Design review of the part built by this model. Coordinates are the model's own, in mm. Face numbers are marked on the shaded views. Coordinates: 2 decimals unless noted, no trailing zeros. Loops run counter-clockwise (first coordinate to the right, second up) from the corner with the lowest first, then second, coordinate; pieces in that order, holes last. Notation, with made-up numbers: (-26.75, -5.75) - (19.25, -5.75) arc R19 cw to (19.25, 22.25) - close; hole circle Ø10 at (5.25, 42.5). An arc over 180 degrees is marked (long way). One line per question, with ' | ' between items.
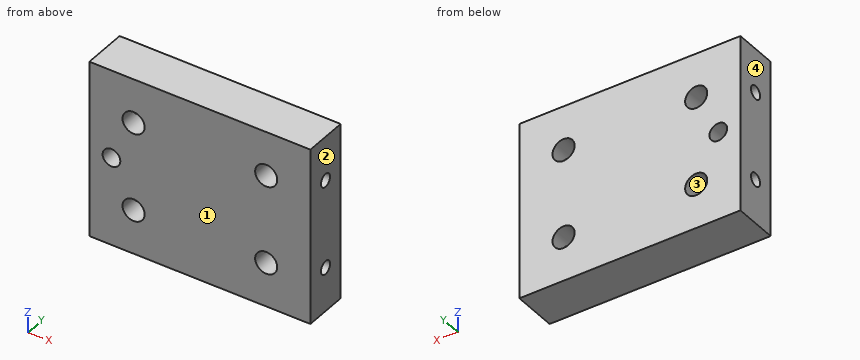
from build123d import *

# Parameters (mm, degrees)
SKETCH_1_W          = 100
SKETCH_1_H          = 80
EXTRUDE_1_DEPTH     = 20
SKETCH_2_R          = 5
SKETCH_2_R_2        = 4
CUT_EXTRUDE_1_DEPTH = 20
SKETCH_3_R          = 3
CUT_EXTRUDE_2_DEPTH = 20
CUT_EXTRUDE_START   = -20
SKETCH_4_R          = 3
CUT_EXTRUDE_3_DEPTH = 20


with BuildPart() as part:
    # Эскиз1 → Бобышка-Вытянуть1 (new body)
    with BuildSketch(Plane(origin=(0, 0, 0), x_dir=(1, 0, 0), z_dir=(0, 1, 0))):
        with Locations((50, 40)):
            Rectangle(SKETCH_1_W, SKETCH_1_H)
    extrude(amount=EXTRUDE_1_DEPTH)

    # Эскиз2 → Вырез-Вытянуть1 (cut)
    with BuildSketch(Plane.XZ):
        with Locations(Location((20, -20, 0), (0, 0, 270))):
            Circle(SKETCH_2_R)
        with Locations(Location((10, -40, 0), (0, 0, 270))):
            Circle(SKETCH_2_R_2)
        with Locations(Location((20, -60, 0), (0, 0, 270))):
            Circle(SKETCH_2_R)
        with Locations(Location((80, -20, 0), (0, 0, 270))):
            Circle(SKETCH_2_R)
        with Locations(Location((80, -60, 0), (0, 0, 270))):
            Circle(SKETCH_2_R)
    extrude(amount=-CUT_EXTRUDE_1_DEPTH, mode=Mode.SUBTRACT)

    # Эскиз3 → Вырез-Вытянуть2 (cut)
    with BuildSketch(Plane.ZY):
        with Locations((-60, 10)):
            Circle(SKETCH_3_R)
        with Locations((-20, 10)):
            Circle(SKETCH_3_R)
    extrude(amount=-CUT_EXTRUDE_2_DEPTH, mode=Mode.SUBTRACT)

    # Эскиз4 → Вырез-Вытянуть3 (cut)
    with BuildSketch(Plane(origin=(100, 0, 0), x_dir=(0, 0, -1), z_dir=(1, 0, 0)).offset(CUT_EXTRUDE_START)):
        with Locations(Location((20, 10, 0), (0, 0, 180))):
            Circle(SKETCH_4_R)
        with Locations(Location((60, 10, 0), (0, 0, 180))):
            Circle(SKETCH_4_R)
    extrude(amount=CUT_EXTRUDE_3_DEPTH, mode=Mode.SUBTRACT)


solid = part.part
Q1. Take a section at C-C (y = 10). Give the boundary of the cut face in (x, z).
Returned:
outline: (0, -80) - (100, -80) - (100, -63) - (84, -63) arc R5 cw (long way) to (84, -57) - (100, -57) - (100, -23) - (84, -23) arc R5 cw (long way) to (84, -17) - (100, -17) - (100, 0) - (0, 0) - (0, -17) - (16, -17) arc R5 cw (long way) to (16, -23) - (0, -23) - (0, -57) - (16, -57) arc R5 cw (long way) to (16, -63) - (0, -63) - close; hole circle Ø8 at (10, -40)
Q2. To check wall thickness, follow line 1 along X through (y, z) = (19.25, -20); line 2 along Y through (x, z) = (94, -60); line 3 along X through (y, z) = (16.5, -24.5). State the ranges of each line that lie inside material, in increasing order.
Returned:
line 1: x = 0 to 15, 25 to 75, 85 to 100 | line 2: y = 0 to 7, 13 to 20 | line 3: x = 0 to 17.82, 22.18 to 77.82, 82.18 to 100
Q3. Take a section at D-D (x = 80). Give the boundary of the cut face in (y, z).
Returned:
outline: (0, -80) - (20, -80) - (20, -65) - (0, -65) - close; (0, -55) - (20, -55) - (20, -25) - (0, -25) - close; (0, -15) - (20, -15) - (20, 0) - (0, 0) - close
Q4. Take a section at A-A (x = 10). Give the boundary of the cut face in (y, z), plus the area to 3 significant figures.
Returned:
outline: (0, -80) - (20, -80) - (20, -44) - (0, -44) - close; (0, -36) - (20, -36) - (20, 0) - (0, 0) - close; hole circle Ø6 at (10, -60); hole circle Ø6 at (10, -20) | area: 1,380 mm²
Q5. Draft analysis for pull direction X (two halves, no side actions). For the marked faces 1, 2, 3 and 4, state which applies: +X half, -X half, draft (parallel to the pull), parting line (faces both ways), or undercut.
Returned:
face 1: draft | face 2: +X half | face 3: undercut | face 4: -X half
Q6. Take a section at B-B (z = -60). Give the boundary of the cut face in (x, y).
Returned:
outline: (0, 0) - (15, 0) - (15, 7) - (0, 7) - close; (0, 13) - (15, 13) - (15, 20) - (0, 20) - close; (25, 0) - (75, 0) - (75, 20) - (25, 20) - close; (85, 0) - (100, 0) - (100, 7) - (85, 7) - close; (85, 13) - (100, 13) - (100, 20) - (85, 20) - close
Q7. For pin 1 (5.5 mm diameter, centred on y = 10, z = -20, fed in from -X); pin 2 (16 mm diameter, centred on x = 80, z = -60, fed in from +Y); pin 3 (5 mm diameter, centred on y = 10, z = -60, fed in from -X); pin 4 (3.5 mm diameter, centred on y = 10, z = -60, fed in from -X), all flat-tipped, find the tip position at first contact; note any pin that passes through.
Returned:
pin 1: stops at x = 24.18 | pin 2: stops at y = 20 | pin 3: stops at x = 24.33 | pin 4: stops at x = 24.68
